Can you work these out from the model? Positions are in its coordinate system, mm. A direction names the side the tool comes from. Give positions to 0.01 mm unless a question says otherwise; leave off trailing zeros. Order: outer loops, then holes, each group sorted by start corner. A loop starts at its lowest first (then second) coordinate and runs counter-clockwise, first axis right, second up. Notation, with made-up numbers: (-32, 53.25) - (-9, 53.25) arc R22 ccw to (-9, 77.25) - close; hole circle Ø5 at (39, 24.5). An arc over 180 degrees is marked (long way). Return JSON: item names as keys, results as strings.
```python
from build123d import *

# Parameters (mm, degrees)
SKETCH1_R                     = 30
BOSS_EXTRUDE1_DEPTH           = 19.125
SKETCH5_W                     = 42
SKETCH5_H                     = 35.5
CUT_EXTRUDE1_DEPTH            = 52.5
SKETCH7_R                     = 11
SKETCH7_W                     = 22
SKETCH7_H                     = 50
CUT_EXTRUDE3_DEPTH            = 52.5
CUT_EXTRUDE4_DEPTH            = 33.25
CBORE_FOR_M4_SHCS1_AT_2_COUNT = 2
CBORE_FOR_M4_SHCS1_AT_2_PITCH = 10


with BuildPart() as part:
    # Sketch1 → Boss-Extrude1 (new, symmetric)
    with BuildSketch(Plane(origin=(0, 0, 0), x_dir=(1, 0, 0), z_dir=(0, 1, 0))):
        with Locations(Location((0, 0, 0), (0, 0, 270))):
            Circle(SKETCH1_R)
    extrude(amount=BOSS_EXTRUDE1_DEPTH, both=True)

    # Sketch5 → Cut-Extrude1 (cut, symmetric)
    with BuildSketch(Plane(origin=(0, 0, 0), x_dir=(0, 0, -1), z_dir=(1, 0, 0))):
        with Locations((9, -1.375)):
            Rectangle(SKETCH5_W, SKETCH5_H)
    extrude(amount=CUT_EXTRUDE1_DEPTH, both=True, mode=Mode.SUBTRACT)

    # Sketch7 → Cut-Extrude3 (cut, symmetric)
    with BuildSketch(Plane(origin=(0, 19.125, 0), x_dir=(1, 0, 0), z_dir=(0, 1, 0))):
        Circle(SKETCH7_R)
        with Locations((0, 25)):
            Rectangle(SKETCH7_W, SKETCH7_H)
    extrude(amount=CUT_EXTRUDE3_DEPTH, both=True, mode=Mode.SUBTRACT)

    # Sketch8 → Cut-Extrude4 (cut)
    with BuildSketch(Plane(origin=(0, 19.125, 0), x_dir=(1, 0, 0), z_dir=(0, 1, 0))):
        with BuildLine():
            Line((10, -28.284271247), (10, -15))
            Line((10, -15), (-10, -15))
            Line((-10, -15), (-10, -28.284271247))
            ThreePointArc((-10, -28.284271247), (-5.073059353, -29.567956791), (1.8e-08, -30))
            ThreePointArc((1.8e-08, -30), (5.07305937, -29.567956788), (10, -28.284271247))
        make_face()
    extrude(amount=-CUT_EXTRUDE4_DEPTH, mode=Mode.SUBTRACT)

    # Sketch11 → CBORE for M4 SHCS1 (revolve, cut)
    with BuildSketch(Plane(origin=(-5, -14.125, 20), x_dir=(0, 0, 1), z_dir=(1, 0, 0))):
        Polygon((0, 0), (0, 7.442065486), (2.4, 6), (2.4, 4), (4, 4), (4, 0.025), (4.025, 0), align=None)
    cbore_for_m4_shcs1 = revolve(axis=Axis((-5, -7.775, 20), (0, -1, 0)), mode=Mode.SUBTRACT)

    # CBORE for M4 SHCS1 at 2: CBORE for M4 SHCS1 ×2
    with Locations(*[(i * CBORE_FOR_M4_SHCS1_AT_2_PITCH, 0, 0) for i in range(1, CBORE_FOR_M4_SHCS1_AT_2_COUNT)]):
        add(cbore_for_m4_shcs1, mode=Mode.SUBTRACT)


solid = part.part
```
1. On a 3-axis mill with a long thin cutter (end or side, diameter ignored), from which of +Z, -Z, +X, -X, +Y, -Y can I reach the whole of each face in a straight line? I mean faces 1 (the face through (0, 18, 11)), 2 (the face through (-3, -18.125, 18)), 3 (the face through (0, -2, 12)), 4 (the face through (10, 3, 22)). Say none if no direction works.
Checks:
{"face 1": "-Z, +Y, -Y", "face 2": "+Y", "face 3": "-Z, +X, -X, -Y", "face 4": "+Z, +Y"}
2. For pin 1 Ø4 at (x, z) = (3, 19) entering from +Y (3 decimals); pin 2 Ø6 at (x, y) = (8, 9) entering from -Z; pin 3 Ø14.5 at (y, z) = (7.5, 20) entering from -X, each with a flat end and sliding along its axis, tell me the tip position at first contact or that it passes through.
Checks:
{"pin 1": "y = -14.125", "pin 2": "z = 12", "pin 3": "x = -27.16"}
3. Suppose I cut it at B-B (z = 20). List the corners of the cut face in (x, y) for me (3 decimals), plus the area to 3 significant figures.
Checks:
{"outline": "(-22.361, -19.125) - (-7.4, -19.125) - (-7.4, -18.125) - (-9, -18.125) - (-9, -14.15) - (-9.025, -14.125) - (-10, -14.125) - (-10, 19.125) - (-22.361, 19.125) - close; (-2.6, -19.125) - (2.6, -19.125) - (2.6, -18.125) - (1, -18.125) - (1, -14.15) - (0.975, -14.125) - (-0.975, -14.125) - (-1, -14.15) - (-1, -18.125) - (-2.6, -18.125) - close; (7.4, -19.125) - (22.361, -19.125) - (22.361, 19.125) - (10, 19.125) - (10, -14.125) - (9.025, -14.125) - (9, -14.15) - (9, -18.125) - (7.4, -18.125) - close", "area": "972 mm^2"}
4. Suppose I cut it at C-C (z = -15). List the corners of the cut face in (x, y) for me (3 decimals).
Checks:
{"outline": "(-25.981, 16.375) - (-11, 16.375) - (-11, 19.125) - (-25.981, 19.125) - close; (11, 16.375) - (25.981, 16.375) - (25.981, 19.125) - (11, 19.125) - close"}
5. If I drill on L1, parallel to X at y = -18, z = 20; L2, parallel to X at y = -18.6, z = 20; L3, parallel to Y at x = 3.5, z = 16 (3 decimals), over which ranges is the centre line in solid material (lowest first)? Write a range as [from, to].
Checks:
{"L1": "[-22.36, -9], [-1, 1], [9, 22.36]", "L2": "[-22.36, -7.4], [-2.6, 2.6], [7.4, 22.36]", "L3": "[-19.125, -14.125]"}
6. Suppose I cut it at D-D (y = 6.5). List the corners of the cut face in (x, z) for me.
Checks:
{"outline": "(-27.5, 12) - (27.5, 12) arc R30 ccw to (10, 28.28) - (10, 15) - (-10, 15) - (-10, 28.28) arc R30 ccw to start"}
7. Suppose I cut it at A-A (x = 0). List the corners of the cut face in (y, z) for me (3 decimals), plus the area to 4 significant figures.
Checks:
{"outline": "(-19.125, 12) - (16.375, 12) - (16.375, 11) - (19.125, 11) - (19.125, 15) - (-14.125, 15) - (-14.125, 30) - (-19.125, 30) - close", "area": "192.5 mm^2"}
8. Thinking about a two-plate mould opening in X: for faces 5 (the face through (-12.31, 2.92, 27.36)), 6 (the face through (-11, 18, -14)), 7 (the face through (14, 16.375, -3)), which applies, +X half, -X half, draft (parallel to the pull), parting line (faces both ways), or undercut?
Checks:
{"face 5": "parting line", "face 6": "undercut", "face 7": "draft"}
